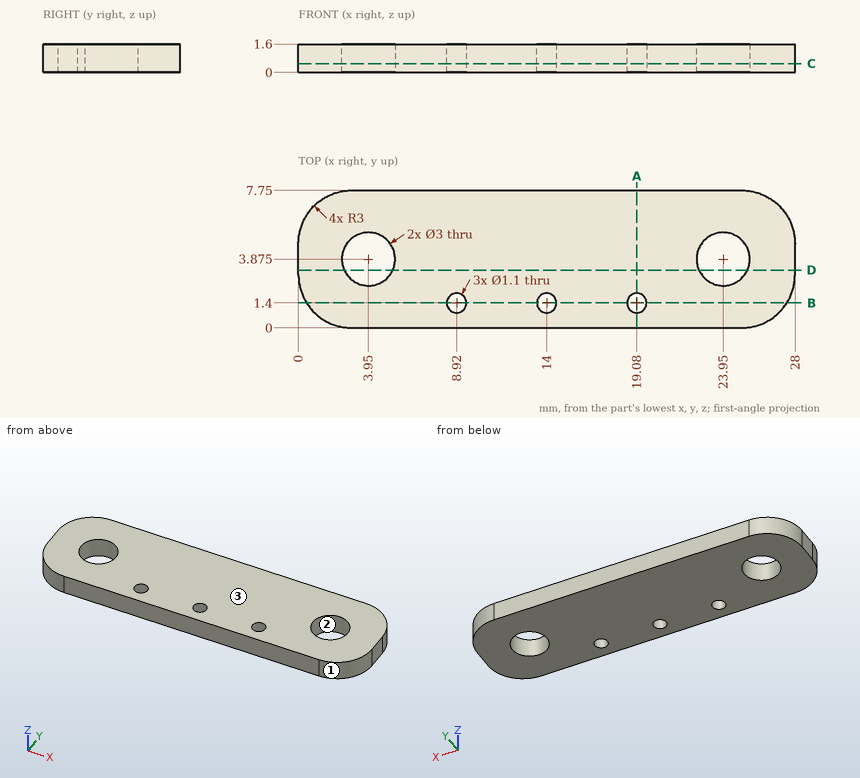
Here's the drawing with two shaded views (mm, measured from the low corner). I have some questions. Round coordinates to 2 decimals unless told otherwise and drop trailing zeros. Write each loop counter-clockwise with the first axis right and the second up, starting at its lowest first coordinate (ties: lowest second). Pieces come first, ordered by that corner, then holes. Notation, with made-up numbers: M 62.25,21 L 91.25,21 A10 cw 91.25,31 Z; hole C 63.25,36.25 d3. An arc over 180 degrees is marked long. Answer in a Markdown table with one row per item. Add a question column.
Q1. If I drill on line 1 (X direction, y = 3.75, z = 0.1); line 2 (Y direction, x = 19.08, z = 0.85); line 3 (Y direction, x = 23.95, z = 0.45) (3 decimals), over which ranges is the centre line in solid material (lowest first)? Write a range as from..to.
Q2. If we mould it in two halves opening along Y, with no side actions, what happens to the marked faces 1, 2 and 3? For each: +Y half, -Y half, draft (parallel to the pull), parting line (faces both ways), or undercut.
Q3. Imagine slicing it at C-C (z = 0.5). Please give me the cut outline in (x, y) (3 decimals).
Q4. Imagine slicing it at A-A (x = 19.08). Please give me the cut outline in (y, z), then the cut area to 3 significant figures.
Q5. Imagine slicing it at B-B (y = 1.4). Please give me the cut outline in (x, z).
Q6. Imagine slicing it at D-D (y = 3.25). Please give me the cut outline in (x, z), then the cut area to 3 significant figures.
Values:
| question | item | result |
|---|---|---|
| 1 | line 1 | 0..2.46, 5.44..22.46, 25.44..28 |
| 1 | line 2 | 0..0.85, 1.95..7.75 |
| 1 | line 3 | 0..2.375, 5.375..7.75 |
| 2 | face 1 | -Y half |
| 2 | face 2 | undercut |
| 2 | face 3 | draft |
| 3 | outline | M 0,3 A3 ccw 3,0 L 25,0 A3 ccw 28,3 L 28,4.75 A3 ccw 25,7.75 L 3,7.75 A3 ccw 0,4.75 Z; hole C 3.95,3.875 d3; hole C 8.92,1.4 d1.1; hole C 14,1.4 d1.1; hole C 19.08,1.4 d1.1; hole C 23.95,3.875 d3 |
| 4 | outline | M 0,0 L 0.85,0 L 0.85,1.6 L 0,1.6 Z; M 1.95,0 L 7.75,0 L 7.75,1.6 L 1.95,1.6 Z |
| 4 | area | 10.6 mm^2 |
| 5 | outline | M 0.46,0 L 8.37,0 L 8.37,1.6 L 0.46,1.6 Z; M 9.47,0 L 13.45,0 L 13.45,1.6 L 9.47,1.6 Z; M 14.55,0 L 18.53,0 L 18.53,1.6 L 14.55,1.6 Z; M 19.63,0 L 27.54,0 L 27.54,1.6 L 19.63,1.6 Z |
| 6 | outline | M 0,0 L 2.59,0 L 2.59,1.6 L 0,1.6 Z; M 5.31,0 L 22.59,0 L 22.59,1.6 L 5.31,1.6 Z; M 25.31,0 L 28,0 L 28,1.6 L 25.31,1.6 Z |
| 6 | area | 36.1 mm^2 |
